```python
from build123d import *

# Parameters (mm, degrees)
ESQUISSE1_W                  = 9
ESQUISSE1_H                  = 45
ESQUISSE1_W_2                = 6
ESQUISSE1_H_2                = 3
BOSS_EXTRU_1_DEPTH           = 2
ENL_V_MAT_EXTRU_1_DEPTH      = 44.887394917
ENL_V_MAT_EXTRU_1_DEPTH_BACK = 44.887394917
ESQUISSE2_W                  = 2.6
ESQUISSE2_H                  = 4.6


with BuildPart() as part:
    # Esquisse1 → Boss.-Extru.1 (new body)
    with BuildSketch(Plane(origin=(0, 0, 0), x_dir=(1, 0, 0), z_dir=(0, 1, 0))):
        with Locations((3.408982136, 20.622516556)):
            Rectangle(ESQUISSE1_W, ESQUISSE1_H)
        with Locations((3.408982136, 35.622516556)):
            Rectangle(ESQUISSE1_W_2, ESQUISSE1_H_2, mode=Mode.SUBTRACT)
        with Locations((3.408982136, 5.622516556)):
            Rectangle(ESQUISSE1_W_2, ESQUISSE1_H_2, mode=Mode.SUBTRACT)
    extrude(amount=BOSS_EXTRU_1_DEPTH)

    # Esquisse2 → Enlèv. mat.-Extru.1 (cut, two sides: drawn at the far end of the back side and taken through both)
    with BuildSketch(Plane.XZ.offset(-ENL_V_MAT_EXTRU_1_DEPTH_BACK)):
        with Locations((3.408982136, -20.622516556)):
            Rectangle(ESQUISSE2_W, ESQUISSE2_H)
    extrude(amount=ENL_V_MAT_EXTRU_1_DEPTH + ENL_V_MAT_EXTRU_1_DEPTH_BACK, mode=Mode.SUBTRACT)


solid = part.part
```
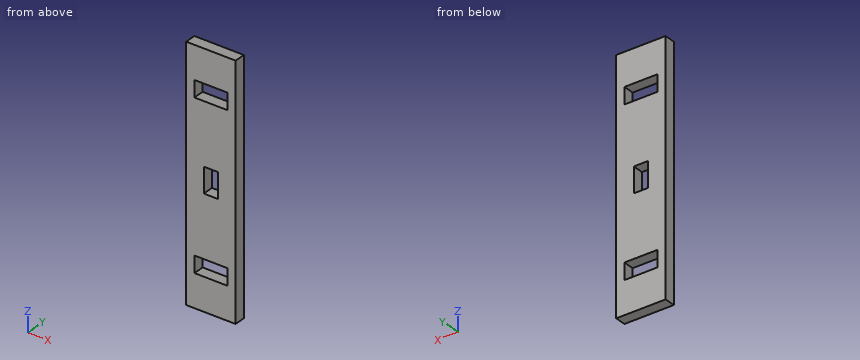
The model under review builds one solid part; all positions refer to its coordinate system, in mm. Coordinates: 2 decimals unless noted, no trailing zeros. Write each loop counter-clockwise with the first axis right and the second up, starting at its lowest first coordinate (ties: lowest second). Pieces come first, ordered by that corner, then holes. Notation, with made-up numbers: (-37, 3.5) -> (12, 3.5) arc R11 ccw to (12, 19.5) -> close; hole circle Ø3 at (49, 51). An arc over 180 degrees is marked (long way). One line per item, written item: value. Start each with the question number.
Q1. Add section D-D, the plane x = 3.5. Give the boundary of the cut face in (y, z).
Q2. Add section C-C, the plane z = -19. Give the boundary of the cut face in (x, y).
Q3. To check wall thickness, follow probe 1 along Z at (x, y) = (2.5, 1.6); probe 2 along Z at (x, y) = (5, 1.8); probe 3 along X at (y, z) = (0.2, -5.5). State the ranges of each line that lie inside material, in increasing order.
Q4. Clearance check with a flat-ended pin moving along its axis: P1, Ø3, axis at x = 4, z = -30, coming from the -Y side. State where the tip first meets the part, or that it passes through.
Q5. Add section A-A, the plane y = 1.1. Give the boundary of the cut face in (x, z), then the cut area to 3 significant figures.
Q6. Add section B-B, the plane x = 1.25. Give the boundary of the cut face in (y, z).
Response:
1. outline: (0, -43.12) -> (2, -43.12) -> (2, -37.12) -> (0, -37.12) -> close; (0, -34.12) -> (2, -34.12) -> (2, -22.92) -> (0, -22.92) -> close; (0, -18.32) -> (2, -18.32) -> (2, -7.12) -> (0, -7.12) -> close; (0, -4.12) -> (2, -4.12) -> (2, 1.88) -> (0, 1.88) -> close
2. outline: (-1.09, 0) -> (2.11, 0) -> (2.11, 2) -> (-1.09, 2) -> close; (4.71, 0) -> (7.91, 0) -> (7.91, 2) -> (4.71, 2) -> close
3. probe 1: -43.12 to -37.12, -34.12 to -22.92, -18.32 to -7.12, -4.12 to 1.88
3. probe 2: -43.12 to -37.12, -34.12 to -7.12, -4.12 to 1.88
3. probe 3: -1.09 to 0.41, 6.41 to 7.91
4. P1: y = 0
5. outline: (-1.09, -43.12) -> (7.91, -43.12) -> (7.91, 1.88) -> (-1.09, 1.88) -> close; hole (0.41, -37.12) -> (6.41, -37.12) -> (6.41, -34.12) -> (0.41, -34.12) -> close; hole (0.41, -7.12) -> (6.41, -7.12) -> (6.41, -4.12) -> (0.41, -4.12) -> close; hole (2.11, -22.92) -> (4.71, -22.92) -> (4.71, -18.32) -> (2.11, -18.32) -> close
5. area: 357 mm²
6. outline: (0, -43.12) -> (2, -43.12) -> (2, -37.12) -> (0, -37.12) -> close; (0, -34.12) -> (2, -34.12) -> (2, -7.12) -> (0, -7.12) -> close; (0, -4.12) -> (2, -4.12) -> (2, 1.88) -> (0, 1.88) -> close
